Job drawing, mm, ordinate dimensions from the low corner. One solid piece. A direction names the side the tool comes from. Round coordinates to 2 decimals unless told otherwise and drop trailing zeros. Order: outer loops, then holes, each group sorted by start corner. A loop starts at its lowest first (then second) coordinate and runs counter-clockwise, first axis right, second up. Notation, with made-up numbers: (49.5, -26) -> (97.5, -26) arc R32 ccw to (97.5, 2) -> close; hole circle Ø3 at (75, -32). An arc over 180 degrees is marked (long way). Return JSON: item names as keys, results as strings. Group by question number.
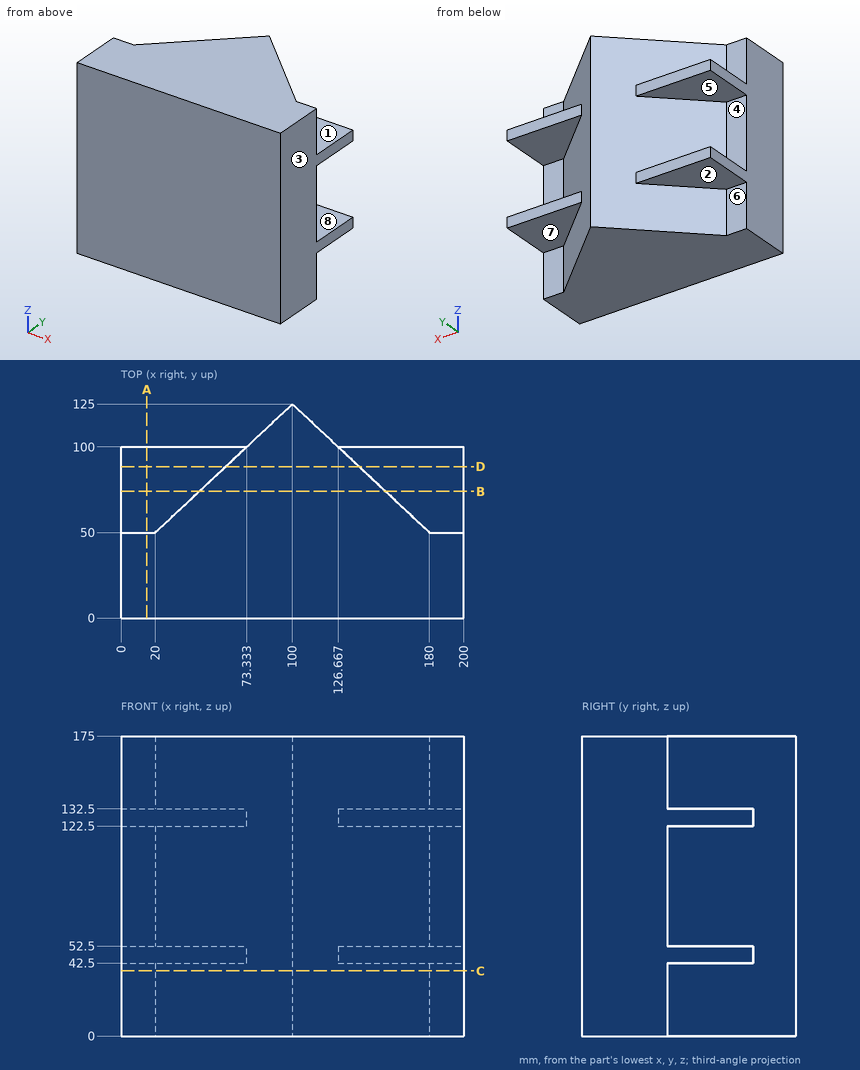
(1) Probe L1, parallel to Z at x = 33, y = 69.5; L2, parallel to Y at x = 189.5, z = 105; L3, parallel to Y at x = 151, z = 97.5. List the from-to ranges inside material, lowest first. Write a range as [from, to].
(2) Pin check, flat tips, straight feed: P1, Ø10, axis at x = 164, z = 46, coming from the -Y side; P2, Ø3, axis at y = 83, z = 72.5, coming from the -X side; P3, Ø16, axis at x = 12.5, z = 18.5, coming from the +Y side; P4, Ø8, axis at x = 26.5, z = 47.5, coming from the +Y side. Stop position of each tip, or through.
(3) Saw through at B-B, the plane y = 74. List the corners of the cut face in (x, z).
(4) Tool access for the marked faces 5, 6, 7 and 8: list every direction of +Z, -Z, +X, -X, +Y, -Y with a clear straight run to the whole face (end or side of a thin tool).
(5) Mould opens along Z. For the marked faces 1, 2, 3 and 4 say: pulls with the +Z half, pulls with the -Z half, needs draft (parallel to the pull), parting line crosses it, or undercut.
(6) Saw through at A-A, the plane x = 15. List the corners of the cut face in (y, z), and give its area (3 significant figures).
(7) Saw through at C-C, the plane z = 38. List the corners of the cut face in (x, y), and give its area (3 significant figures).
(8) Saw through at D-D, the plane y = 88.5. List the corners of the cut face in (x, z).
Results are:
{
 "1": {"L1": "z = [42.5, 52.5], [122.5, 132.5]", "L2": "y = [0, 50]", "L3": "y = [0, 77.19]"},
 "2": {"P1": "stops at y = 0", "P2": "stops at x = 53.6", "P3": "stops at y = 50.47", "P4": "stops at y = 100"},
 "3": {"outline": "(0, 42.5) -> (45.6, 42.5) -> (45.6, 0) -> (154.4, 0) -> (154.4, 42.5) -> (200, 42.5) -> (200, 52.5) -> (154.4, 52.5) -> (154.4, 122.5) -> (200, 122.5) -> (200, 132.5) -> (154.4, 132.5) -> (154.4, 175) -> (45.6, 175) -> (45.6, 132.5) -> (0, 132.5) -> (0, 122.5) -> (45.6, 122.5) -> (45.6, 52.5) -> (0, 52.5) -> close"},
 "4": {"face 5": "-X, +Y", "face 6": "-Z, -X, +Y", "face 7": "-Z, +X, +Y", "face 8": "+X, +Y"},
 "5": {"face 1": "pulls with the +Z half", "face 2": "pulls with the -Z half", "face 3": "needs draft", "face 4": "undercut"},
 "6": {"outline": "(0, 0) -> (50, 0) -> (50, 42.5) -> (100, 42.5) -> (100, 52.5) -> (50, 52.5) -> (50, 122.5) -> (100, 122.5) -> (100, 132.5) -> (50, 132.5) -> (50, 175) -> (0, 175) -> close", "area": "9,750 mm^2"},
 "7": {"outline": "(0, 0) -> (200, 0) -> (200, 50) -> (180, 50) -> (100, 125) -> (20, 50) -> (0, 50) -> close", "area": "16,000 mm^2"},
 "8": {"outline": "(0, 42.5) -> (61.07, 42.5) -> (61.07, 0) -> (138.93, 0) -> (138.93, 42.5) -> (200, 42.5) -> (200, 52.5) -> (138.93, 52.5) -> (138.93, 122.5) -> (200, 122.5) -> (200, 132.5) -> (138.93, 132.5) -> (138.93, 175) -> (61.07, 175) -> (61.07, 132.5) -> (0, 132.5) -> (0, 122.5) -> (61.07, 122.5) -> (61.07, 52.5) -> (0, 52.5) -> close"}
}
